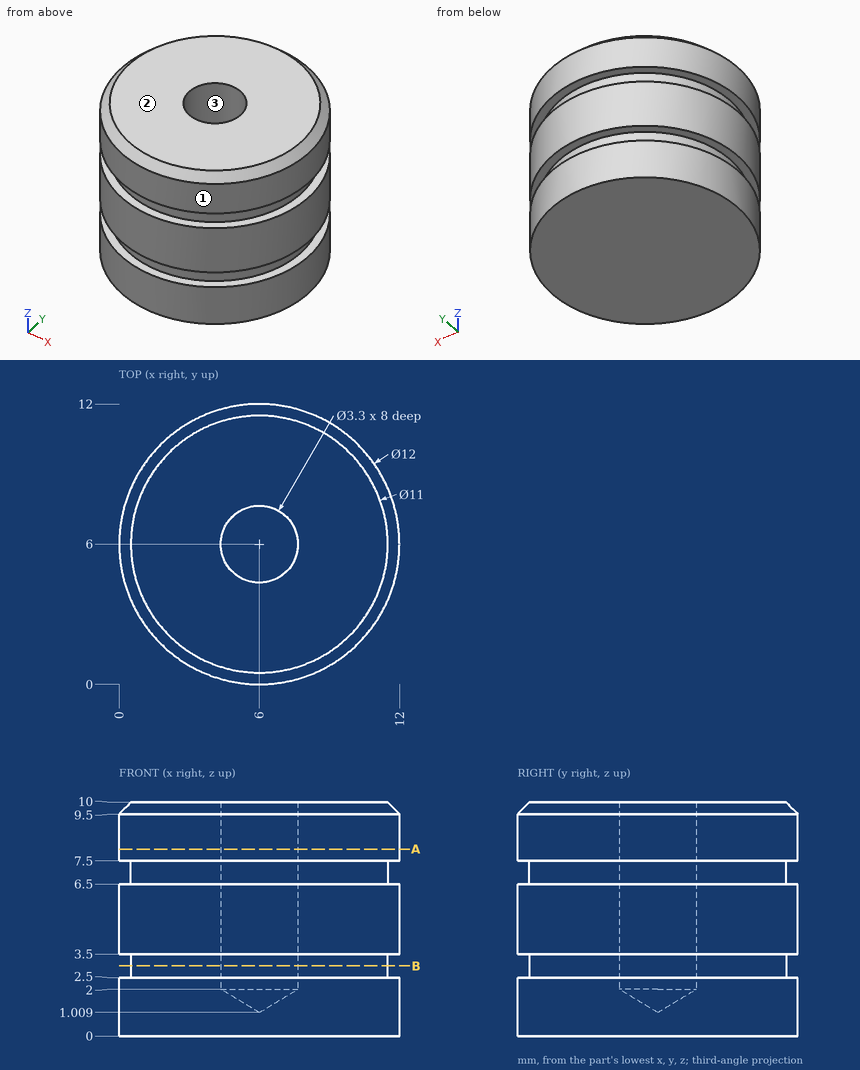
Here's the drawing with two shaded views (mm, measured from the low corner). I have some questions. Coordinates: 2 decimals unless noted, no trailing zeros. Order: outer loops, then holes, each group sorted by start corner. A loop starts at its lowest first (then second) coordinate and runs counter-clockwise, first axis right, second up.
Q1. Will these pins go through, and if not, where does the flat tip stop? pin 1 (5 mm diameter, centred on y = 2, z = 7, fed in from +X); pin 2 (2 mm diameter, centred on y = 6.5, z = 2.5, fed in from +X).
Q2. Suppose I cut it at A-A on z = 8. Please give me the cut outline in (x, y).
Q3. Thinking about a two-plate mould opening in X: for the marked faces 1, 2 and 3, which applies, released by +X, released by -X, zero draft, split by the parting line, or undercut?
Q4. Please list where these lines run through material, in increasing order: L1, parallel to Y at x = 6, z = 7.25; L2, parallel to Y at x = 6, z = 4; L3, parallel to Y at x = 10.5, z = 1.
Q5. Suppose I cut it at B-B on z = 3. Please give me the cut outline in (x, y).
Answer:
1. pin 1: stops at x = 11.8
1. pin 2: stops at x = 12
2. outline: circle Ø12 at (6, 6); hole circle Ø3.3 at (6, 6)
3. face 1: split by the parting line
3. face 2: zero draft
3. face 3: undercut
4. L1: y = 0.5 to 4.35, 7.65 to 11.5
4. L2: y = 0 to 4.35, 7.65 to 12
4. L3: y = 2.03 to 9.97
5. outline: circle Ø11 at (6, 6); hole circle Ø3.3 at (6, 6)
